For this review, take the finished solid that the model builds, in its own axes (mm). A direction names the side the tool comes from. Coordinates: 2 decimals unless noted, no trailing zeros. Loops run counter-clockwise (first coordinate to the right, second up) from the corner with the lowest first, then second, coordinate; pieces in that order, holes last. Notation, with made-up numbers: M 40,55 L 53,55 A21 ccw 53,82 Z; hole C 33.25,2 d11. An arc over 180 degrees is marked long. Write item = value, one per line.
from build123d import *

# Parameters (mm, degrees)
SKETCH_R             = 8.6
PAD_DEPTH            = 1
SKETCH001_R          = 8.6
SKETCH001_R_2        = 3.2
PAD001_DEPTH         = 6.6
SKETCH002_W          = 2
SKETCH002_H          = 2
POCKET_DEPTH         = 8.601
POCKET_DEPTH_BACK    = -8.601
SKETCH003_R          = 8.6
SKETCH003_R_2        = 8.1
PAD002_DEPTH         = 36
SKETCH004_W          = 6
SKETCH004_H          = 4
POCKET001_DEPTH      = 8.601
POCKET001_DEPTH_BACK = -8.601


with BuildPart() as part:
    # Sketch → Pad (new body)
    with BuildSketch(Plane.XY):
        Circle(SKETCH_R)
    extrude(amount=PAD_DEPTH)

    # Sketch001 (on Face3 of Pad) → Pad001 (join)
    with BuildSketch(Plane.XY.offset(1)):
        Circle(SKETCH001_R)
        Circle(SKETCH001_R_2, mode=Mode.SUBTRACT)
    extrude(amount=PAD001_DEPTH)

    # Sketch002 → Pocket (cut, two sides)
    with BuildSketch(Plane.XZ) as pocket_sk:
        with Locations((0, 2)):
            Rectangle(SKETCH002_W, SKETCH002_H)
    extrude(amount=-POCKET_DEPTH, mode=Mode.SUBTRACT)
    extrude(pocket_sk.sketch, amount=-POCKET_DEPTH_BACK, mode=Mode.SUBTRACT)

    # Sketch003 (on Face12 of Pocket) → Pad002 (join)
    with BuildSketch(Plane.XY.offset(7.6)):
        Circle(SKETCH003_R)
        Circle(SKETCH003_R_2, mode=Mode.SUBTRACT)
    extrude(amount=PAD002_DEPTH)

    # Sketch004 → Pocket001 (cut, two sides)
    with BuildSketch(Plane.XZ) as pocket001_sk:
        with Locations((0, 38.6)):
            Rectangle(SKETCH004_W, SKETCH004_H)
    extrude(amount=-POCKET001_DEPTH, mode=Mode.SUBTRACT)
    extrude(pocket001_sk.sketch, amount=-POCKET001_DEPTH_BACK, mode=Mode.SUBTRACT)


solid = part.part
Q1. Add section C-C (z = 5). Write out the cut boundary in (x, y).
Solved:
outline = C 0,0 d17.2; hole C 0,0 d6.4
Q2. Add section A-A (x = 0). Write out the cut boundary in (y, z).
Solved:
outline = M -8.6,0 L 8.6,0 L 8.6,1 L -8.6,1 Z; M -8.6,3 L -3.2,3 L -3.2,7.6 L -8.1,7.6 L -8.1,36.6 L -8.6,36.6 Z; M -8.6,40.6 L -8.1,40.6 L -8.1,43.6 L -8.6,43.6 Z; M 3.2,3 L 8.6,3 L 8.6,36.6 L 8.1,36.6 L 8.1,7.6 L 3.2,7.6 Z; M 8.1,40.6 L 8.6,40.6 L 8.6,43.6 L 8.1,43.6 Z
Q3. Add section B-B (y = 0). Write out the cut boundary in (x, z).
Solved:
outline = M -8.6,0 L 8.6,0 L 8.6,43.6 L 8.1,43.6 L 8.1,7.6 L 3.2,7.6 L 3.2,1 L -3.2,1 L -3.2,7.6 L -8.1,7.6 L -8.1,43.6 L -8.6,43.6 Z
Q4. For pin 1 Ø1.9 at (x, y) = (1.5, -2) entering from +Z; pin 2 Ø4 at (x, y) = (0, 0) entering from +Z; pin 3 Ø1.6 at (y, z) = (-6.5, 2) entering from -X, all flat-tipped, find the tip position at first contact; note any pin that passes through.
Solved:
pin_1 = 7.6
pin_2 = 1
pin_3 = -6.44
Q5. Add section D-D (y = -5.75). Write out the cut boundary in (x, z).
Solved:
outline = M -6.4,0 L 6.4,0 L 6.4,43.6 L 5.71,43.6 L 5.71,7.6 L -5.71,7.6 L -5.71,43.6 L -6.4,43.6 Z; hole M -1,1 L 1,1 L 1,3 L -1,3 Z
Q6. Machinability: for faces 4 (the face through (0, 0, 0)), 5 (the face through (3.5, 0.1, 7.6)), 6 (the face through (0, 0, 1)), 7 (the face through (-1, 6, 2)), which of the approach directions +Z, -Z, +X, -X, +Y, -Y give a long, thin tool a straight path to every point of the face, cutting with its end or side? Answer none if there is none.
Solved:
face_4 = -Z, +X, -X, +Y, -Y
face_5 = +Z
face_6 = none
face_7 = +Y, -Y
Q7. Draft analysis for pull direction Y (two halves, no side actions). For faces 1 (the face through (-8.59, 0.38, 21.49)), 2 (the face through (1, 6, 2)), 3 (the face through (7.726, 2.433, 25.348)), state which applies: +Y half, -Y half, draft (parallel to the pull), parting line (faces both ways), or undercut.
Solved:
face_1 = parting line
face_2 = draft
face_3 = undercut
Q8. For line 1 along Y through (x, z) = (0, 26); line 2 along Y through (x, z) = (0, 4.25); line 3 along Z through (x, y) = (-7.5, -0.25), list the stretches that pass through material, from the lowest coordinate up.
Solved:
line_1 = -8.6 to -8.1, 8.1 to 8.6
line_2 = -8.6 to -3.2, 3.2 to 8.6
line_3 = 0 to 7.6
